Model file for the job. Use its own axes, mm. A direction names the side the tool comes from. Give positions to 0.01 mm unless a question says otherwise; leave off trailing zeros. Write each loop counter-clockwise with the first axis right and the second up, starting at its lowest first coordinate (ties: lowest second). Pieces come first, ordered by that corner, then holes. Notation, with made-up numbers: (-23.75, 86) - (17.25, 86) arc R24 ccw to (17.25, 119) - close; hole circle Ø1 at (-25, 27.25). An arc over 180 degrees is marked (long way). Use CSV: the item, a comma, the result in double quotes.
from build123d import *

# Parameters (mm, degrees)
F2_T = -2.5


with BuildPart() as f1:
    # F0 (on Right) → F1 (revolve)
    with BuildSketch(Plane.YZ):
        Polygon((-21.9740401953, -59.7611889243), (0, -59.7611889243), (0, 60.1719170809), (-39.6354235709, 60.1719170809), (-39.6354235709, 38.8139672577), (-21.9740401953, 19.9203956872), align=None)
    revolve(axis=Axis((0, 0, 0.2053640783), (0, 0, -1)))

    # F2
    f2_openings = [f1.faces().sort_by_distance(p)[0] for p in [
        (0, 0, 60.171917),
    ]]
    offset(amount=F2_T, openings=f2_openings, kind=Kind.INTERSECTION)


solid = f1.part
(1) Saw through at A-A, the plane y = 0. List the corners of the cut face in (x, z), then the cut area to 3 significant figures.
Checked values:
outline,"(-39.64, 38.81) - (-21.97, 19.92) - (-21.97, -59.76) - (21.97, -59.76) - (21.97, 19.92) - (39.64, 38.81) - (39.64, 60.17) - (37.14, 60.17) - (37.14, 39.8) - (19.47, 20.91) - (19.47, -57.26) - (-19.47, -57.26) - (-19.47, 20.91) - (-37.14, 39.8) - (-37.14, 60.17) - (-39.64, 60.17) - close"
area,"732 mm^2"
(2) 3-axis set-ups, long thin cutter, end or side, ignore diameter. For faces 4 (the face through (0, 0, -59.761)), 5 (the face through (-11.15, -35.42, 49.84)): which of +Z, -Z, +X, -X, +Y, -Y reach the whole face in a straight line?
Checked values:
face 4,"-Z, +X, -X, +Y, -Y"
face 5,"+Z"
(3) Pull direction X, two halves, no side cores. Call faces 1 (the face through (21.452, 4.764, -20.478)), 2 (the face through (-35.4, -11.9, 60.172)), 3 (the face through (-6.11, -19.39, 21.82)): released by +X, released by -X, zero draft, split by the parting line, or undercut.
Checked values:
face 1,"split by the parting line"
face 2,"zero draft"
face 3,"undercut"
(4) Saw through at B-B, the plane z = -3. List the corners of the cut face in (x, y).
Checked values:
outline,"circle Ø43.95 at (0, 0); hole circle Ø38.95 at (0, 0)"
(5) Saw through at D-D, the plane z = 33. List the corners of the cut face in (x, y), then the cut area to 3 significant figures.
Checked values:
outline,"circle Ø68.4 at (0, 0); hole circle Ø61.56 at (0, 0)"
area,"699 mm^2"
(6) Wall check: probe 1 along X at (y, z) = (0, -33); probe 2 along Y at (x, z) = (0, 52.25). Give the ranges that are in metal, low to high. Write a range as [from, to].
Checked values:
probe 1,"x = [-21.97, -19.47], [19.47, 21.97]"
probe 2,"y = [-39.64, -37.14], [37.14, 39.64]"
(7) Flat gauge pins, fed straight in: P1, Ø4, axis at y = -25.5, z = 27.5, coming from the -X side; P2, Ø12, axis at y = 23.5, z = 14, coming from the -X side; P3, Ø6, axis at x = -11.5, y = -19, coming from the +Z side. Where does each tip first touch, or does it go through?
Checked values:
P1,"stops at x = -18.53"
P2,"stops at x = -13.29"
P3,"stops at z = 27.04"
